The figure shows three views and two pictorial views of one solid part (mm, origin at its lowest corner). Answer the questions. Coordinates: 2 decimals unless noted, no trailing zeros. Write each loop counter-clockwise with the first axis right and the second up, starting at its lowest first coordinate (ties: lowest second). Pieces come first, ordered by that corner, then holes.
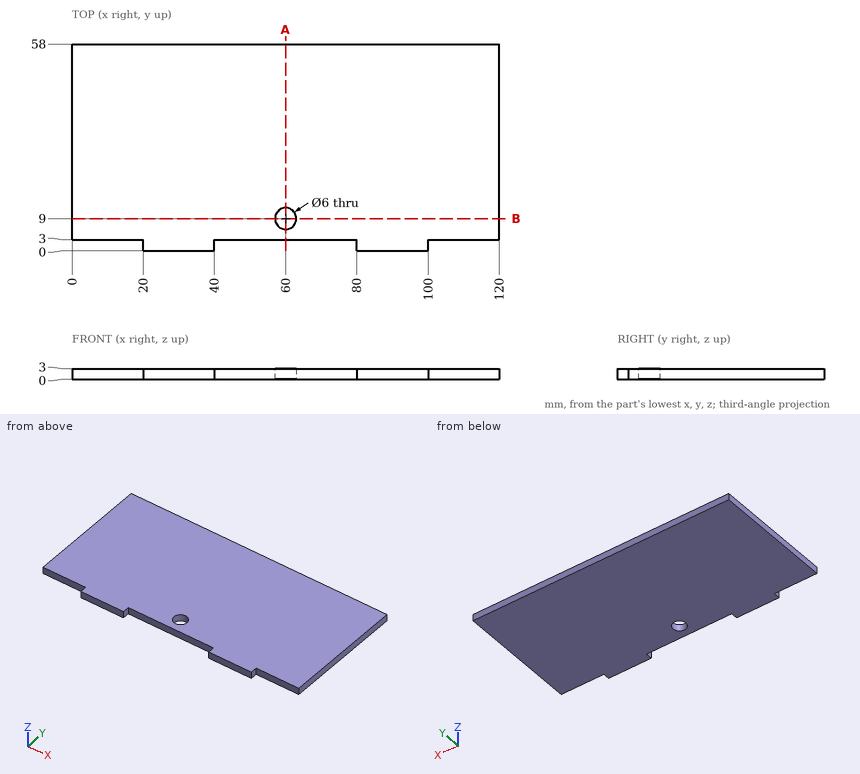
Item 1: The part is cut by section A-A (x = 60). Give the vertices of the cut face in (y, z), and give its area (3 significant figures).
Item 2: Find the intervals of material crossed by probe 1 along Y at (x, z) = (60, 2.2); probe 2 along Y at (x, z) = (8, 2.95), in increasing order.
Item 3: Given pin 1 (1.5 mm diameter, centred on y = 2, z = 1.5, fed in from +X); pin 2 (0.9 mm diameter, centred on x = 9, z = 1.5, fed in from -Y); pin 3 (0.9 mm diameter, centred on y = 2, z = 1, fed in from -X), each flat-ended and moving along its own axis, determine where each tip first touches the part or whether it passes through.
Item 4: The part is cut by section B-B (y = 9). Give the vertices of the cut face in (x, z).
Answer:
1. outline: (3, 0) - (6, 0) - (6, 3) - (3, 3) - close; (12, 0) - (58, 0) - (58, 3) - (12, 3) - close
1. area: 147 mm2
2. probe 1: y = 3 to 6, 12 to 58
2. probe 2: y = 3 to 58
3. pin 1: stops at x = 100
3. pin 2: stops at y = 3
3. pin 3: stops at x = 20
4. outline: (0, 0) - (57, 0) - (57, 3) - (0, 3) - close; (63, 0) - (120, 0) - (120, 3) - (63, 3) - close
